```python
from build123d import *

# Parameters (mm, degrees)
CYLINDER_R        = 1
CYLINDER_DEPTH    = 40
CYLINDER001_R     = 1
CYLINDER001_DEPTH = 10
FILLET_R          = 0.5


with BuildPart() as esfera:
    # Sphere → Sphere (revolve)
    with BuildSketch(Plane(origin=(0, 0, 32.2), x_dir=(1, 0, 0), z_dir=(0, -1, 0))):
        with BuildLine():
            ThreePointArc((0, -3.5), (3.5, 0), (0, 3.5))
            Line((0, 3.5), (0, -3.5))
        make_face()
    revolve(axis=Axis((0, 0, 32.2), (0, 0, 1)))


with BuildPart() as cono:
    # Cone → Cone (revolve)
    with BuildSketch(Plane(origin=(0, 0, 28), x_dir=(1, 0, 0), z_dir=(0, -1, 0))):
        Polygon((0, 0), (1, 0), (3, 3), (0, 3), align=None)
    revolve(axis=Axis((0, 0, 28), (0, 0, 1)))


with BuildPart() as fusion:
    # Cylinder → Cylinder (new body)
    with BuildSketch(Plane.XY.offset(-12)):
        Circle(CYLINDER_R)
    extrude(amount=CYLINDER_DEPTH)

    # Fusion: union Cono
    add(cono.part)


with BuildPart() as fusion002:
    # Cylinder001 → Cylinder001 (new body)
    with BuildSketch(Plane.XY.offset(25.8)):
        Circle(CYLINDER001_R)
    extrude(amount=CYLINDER001_DEPTH)

    # Fillet
    fillet_edges = [fusion002.edges().sort_by_distance(p)[0] for p in [
        (-1, 0, 35.8),
    ]]
    fillet(fillet_edges, radius=FILLET_R)

    # Fusion001: union Fusion
    add(fusion.part)

    # Fusion002: union Esfera
    add(esfera.part)


solid = fusion002.part
```
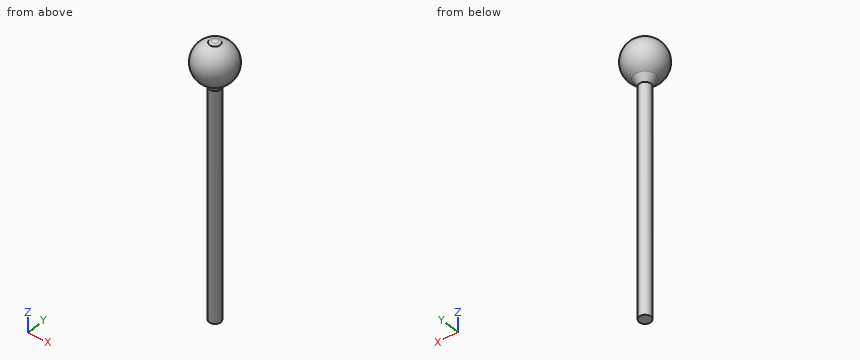
Could you check a few things on this model? Use its own coordinates, in mm. Give positions to 0.01 mm unless a question says otherwise; leave off trailing zeros. Order: outer loops, then holes, each group sorted by start corner. A loop starts at its lowest first (then second) coordinate and runs counter-clockwise, first axis right, second up.
Q1. If I drill on line 1 along Y through (x, z) = (0, 25); line 2 along Z through (x, y) = (-2.25, 2); line 3 along Z through (x, y) = (1, -3), over which ranges is the centre line in solid material (lowest first)?
Q2. Suppose I cut it at B-B, the plane x = 2.5. Write out the boundary of the cut face in (y, z).
Q3. Suppose I cut it at A-A, the plane z = 23. Write out the boundary of the cut face in (x, y), and give its area (3 significant figures).
Q4. I'm going to push flat-ended pins straight in: P1, Ø1.5, axis at y = 1.5, z = 8, coming from the +X side; P2, Ø4, axis at y = 1.5, z = 16, coming from the -X side; P3, Ø1, axis at x = 0, z = 28, coming from the -Y side. Where does each tip first touch, or does it pass through?
Solution:
1. line 1: y = -1 to 1
1. line 2: z = 30.41 to 33.99
1. line 3: z = 30.7 to 33.7
2. outline: circle Ø4.9 at (0, 32.2)
3. outline: circle Ø2 at (0, 0)
3. area: 3.14 mm2
4. P1: stops at x = 0.66
4. P2: stops at x = -1
4. P3: stops at y = -1.33
